Autodesk Inventor part; units mm, degrees
ref_plane "Work Plane5" through (-11.5, 0, 1.25) normal (1, 0, 0) x (0, 0, -1)
ref_plane "Work Plane6" through (-24.25, 0, -17.5) normal (0, 0, 1) x (1, 0, 0)
ref_plane "YZ Plane" through (0, 0, 0) normal (1, 0, 0) x (0, 1, 0)
sketch "Sketch1" plane through (0, 0, 0) normal (0, 1, 0) x (-1, 0, 0)
  line L0 (0, 0) -> (23, 0) construction
  line L1 (23, 0) -> (23, -35) construction
  line L2 (23, -35) -> (0, -35) construction
  line L3 (0, -35) -> (0, 0) construction
  line L4 (23.25, -35.25) -> (23.25, 0.25)
  line L5 (23.25, 0.25) -> (-0.25, 0.25)
  line L6 (-0.25, 0.25) -> (-0.25, -35.25)
  line L7 (-0.25, -35.25) -> (23.25, -35.25)
  line L8 (24.25, 1.25) -> (24.25, -36.25)
  line L9 (24.25, -36.25) -> (-1.25, -36.25)
  line L10 (-1.25, -36.25) -> (-1.25, 1.25)
  line L11 (-1.25, 1.25) -> (24.25, 1.25)
  dimension "d0" = 35
  dimension "d1" = 23
  dimension "d2" = 0.25
  dimension "d3" = 1
extrude "Extrusion1" add sketch "Sketch1" along normal blind 8
sketch "Sketch9" plane through (0.25, 0, 0.25) normal (0, 0, -1) x (-1, 0, 0)
  line L0 (-1, 0) -> (24.5, 0)
  line L1 (24.5, 0) -> (24.5, 8)
  line L2 (-1, 8) -> (24.5, 8)
  line L3 (-1, 0) -> (-1, 8)
  line L4 (0, 0) -> (23.5, 0)
  line L5 (23.5, 0) -> (23.5, 8)
  line L6 (0, 8) -> (23.5, 8)
  line L7 (0, 0) -> (0, 8)
  line L8 (0, 8) -> (3, 8)
  line L9 (24.5, 8) -> (-1, 8)
  line L10 (3, 8) -> (0, 5.5)
  line L11 (0, 0) -> (0, 8)
  line L12 (0, 8) -> (0, 5.5)
  point P0 (0.25, 0)
  point P1 (0, 8)
  dimension "d25" = 3
  dimension "d26" = 2.5
extrude "Extrusion7" add sketch "Sketch9" along normal up to surface (35.5 mm away) contours L7 L2 L10
ref_plane "Work Plane5" through (-11.5, 0, 1.25) normal (1, 0, 0) x (0, 0, -1)
mirror "Mirror4" about plane through (-11.5, 0, 1.25) normal (1, 0, 0) of "Extrusion7"
sketch "Sketch10" plane through (0.25, 0, -35.25) normal (-1, 0, 0) x (0, 0, 1)
  line L0 (-1, 0) -> (36.5, 0)
  line L1 (36.5, 0) -> (36.5, 8)
  line L2 (-1, 8) -> (36.5, 8)
  line L3 (-1, 0) -> (-1, 8)
  line L4 (35.5, 5.5) -> (0, 5.5)
  line L5 (0, 0) -> (0, 5.5)
  line L6 (0, 0) -> (35.5, 0)
  line L7 (35.5, 0) -> (35.5, 5.5)
  line L8 (36.5, 8) -> (-1, 8)
  line L9 (0, 8) -> (3, 8)
  line L10 (0, 0) -> (0, 5.5)
  line L11 (3, 8) -> (0, 5.5)
  line L12 (35.5, 5.5) -> (0, 5.5)
  line L13 (0, 8) -> (0, 5.5)
  point P0 (35.25, 0)
  point P1 (3, 8)
  dimension "d29" = 3
extrude "Extrusion8" add sketch "Sketch10" along normal up to surface (23.5 mm away) contours L13 L2 L11
ref_plane "Work Plane6" through (-24.25, 0, -17.5) normal (0, 0, 1) x (1, 0, 0)
mirror "Mirror5" about plane through (-24.25, 0, -17.5) normal (0, 0, 1) of "Extrusion8"
sketch "Sketch11" plane through (0, 8, 0) normal (0, 1, 0) x (1, 0, 0)
  line L0 (1.25, -1.25) -> (1.25, 36.25)
  line L1 (-24.25, -1.25) -> (1.25, -1.25)
  line L2 (-24.25, 36.25) -> (-24.25, -1.25)
  line L3 (1.25, 36.25) -> (-24.25, 36.25)
  line L4 (-23.25, 35.25) -> (0.25, 35.25)
  line L5 (-23.25, -0.25) -> (-23.25, 35.25)
  line L6 (0.25, -0.25) -> (-23.25, -0.25)
  line L7 (0.25, 35.25) -> (0.25, -0.25)
  point P0 (0, 0)
extrude "Extrusion9" add sketch "Sketch11" along normal blind 3
sketch "Sketch12" plane through (-23.25, 0, -35.25) normal (0, 0, 1) x (1, 0, 0)
  line L0 (23.5, 5.5) -> (0, 5.5)
  line L1 (0, 0) -> (0, 5.5)
  line L2 (0, 0) -> (23.5, 0)
  line L3 (23.5, 0) -> (23.5, 5.5)
  line L4 (0, 5.5) -> (15, 5.5)
  line L5 (15, 5.5) -> (15, 3.5)
  line L6 (15, 3.5) -> (0, 3.5)
  line L7 (0, 3.5) -> (0, 5.5)
  point P0 (23.25, 0)
  point P1 (0, 5.5)
  point P2 (0, 3.5)
  dimension "d34" = 3.5
  dimension "d35" = 2
  dimension "d36" = 15
extrude "Extrusion10" add sketch "Sketch12" along normal blind 3 contours L5 L6 L1 L0
sketch "Sketch13" plane through (0.25, 0, 0.25) normal (0, 0, -1) x (-1, 0, 0)
  line L0 (23.5, 3.5) -> (23.5, 5.5)
  line L1 (8.5, 5.5) -> (23.5, 5.5)
  line L2 (8.5, 3.5) -> (23.5, 3.5)
  line L3 (23.5, 0) -> (23.5, 3.5)
  line L4 (23.5, 0) -> (0, 0)
  line L5 (0, 0) -> (0, 5.5)
  line L6 (0, 5.5) -> (8.5, 5.5)
  line L7 (8.5, 5.5) -> (8.5, 3.5)
  line L8 (7.5, 5.5) -> (7.5, 3.5)
  line L9 (7.5, 3.5) -> (3.5, 3.5)
  line L10 (3.5, 3.5) -> (3.5, 5.5)
  line L11 (3.5, 5.5) -> (7.5, 5.5)
  line L12 (21.5, 5.5) -> (23.5, 5.5)
  line L13 (23.5, 5.5) -> (23.5, 3.5)
  line L14 (23.5, 3.5) -> (21.5, 3.5)
  line L15 (21.5, 3.5) -> (21.5, 5.5)
  point P0 (0.25, 0)
  dimension "d40" = 4
  dimension "d41" = 2
  dimension "d42" = 3.5
  dimension "d49" = 2
extrude "Extrusion11" add sketch "Sketch13" along normal blind 2 contours L2 L15 L1 L0 | L8 L9 L10 L6
sketch "Sketch18" plane through (-23.25, 5.5, -35.25) normal (0, 1, 0) x (1, 0, 0)
  line L0 (16, -35.5) -> (20, -35.5)
  line L1 (20, -35.5) -> (20, -33.5)
  line L2 (16, -33.5) -> (20, -33.5)
  line L3 (16, -35.5) -> (16, -33.5)
  line L4 (0, -35.5) -> (2, -35.5)
  line L5 (2, -35.5) -> (2, -33.5)
  line L6 (0, -33.5) -> (2, -33.5)
  line L7 (0, -33.5) -> (0, -35.5)
  line L8 (15, 0) -> (0, 0)
  line L9 (0, 0) -> (0, -3)
  line L10 (15, -3) -> (0, -3)
  line L11 (15, 0) -> (15, -3)
  point P0 (23.25, -35.25)
extrude "Extrusion14" add sketch "Sketch18" along normal up to surface (2.5 mm away)
sketch "Sketch20" plane through (-23.25, 3.5, -35.25) normal (0, -1, 0) x (1, 0, 0)
  line L0 (0, 35.5) -> (2, 35.5)
  line L1 (0, 33.5) -> (0, 35.5)
  line L2 (2, 33.5) -> (0, 33.5)
  line L3 (2, 35.5) -> (2, 33.5)
  line L4 (16, 35.5) -> (20, 35.5)
  line L5 (16, 35.5) -> (16, 33.5)
  line L6 (20, 33.5) -> (16, 33.5)
  line L7 (20, 35.5) -> (20, 33.5)
  line L8 (15, 0) -> (0, 0)
  line L9 (15, 0) -> (15, 3)
  line L10 (0, 3) -> (15, 3)
  line L11 (0, 0) -> (0, 3)
  point P0 (23.25, 35.25)
extrude "Extrusion16" cut sketch "Sketch20" against normal blind 0.5
sketch "Sketch22" plane through (-23.25, 0, -35.25) normal (0, 0, 1) x (1, 0, 0)
  point P0 (23.25, 0)
sketch "Sketch23" plane through (-23.25, 0, -35.25) normal (0, 0, 1) x (1, 0, 0)
  point P0 (23.25, 0)
properties part number "sensorCover"
The model under review builds one solid part; all positions refer to its coordinate system, in mm. A direction names the side the tool comes from. Give positions to 0.01 mm unless a question says otherwise; leave off trailing zeros. Write each loop counter-clockwise with the first axis right and the second up, starting at its lowest first coordinate (ties: lowest second). Pieces come first, ordered by that corner, then holes. Notation, with made-up numbers: M 24,75.5 L 54,75.5 A14 ccw 54,94.5 Z; hole C 88.25,41 d2. An arc over 180 degrees is marked long. One line per question, with ' | ' between items. Start each with the question number.
Item 1: We need section A-A on z = -7. Write out the cut boundary in (x, y).
Item 2: Wall thickness on line 1 (X direction, y = 0.75, z = -1); line 2 (Z direction, x = -7.5, y = 2.5); line 3 (X direction, y = 4.5, z = -1): over which ranges is each line inside the solid? List them lowest first. Write a range as from..to.
Item 3: We need section C-C on x = -16. Write out the cut boundary in (y, z), plus the area to 4 significant figures.
Item 4: Draft analysis for pull direction X (two halves, no side actions). For faces 3 (the flat face through (-24.25, 5, -18)), 4 (the flat face through (1.25, 5, -17)), 5 (the flat face through (-11, 2, -35.25)), state which applies: released by +X, released by -X, zero draft, split by the parting line, or undercut.
Item 5: We need section D-D on y = 4.5. Write out the cut boundary in (x, z).
Item 6: For faces 1 (the flat face through (-22, 4, -1)), 2 (the flat face through (-23.25, 9, -17)), list the 3-axis set-ups (+Z, -Z, +X, -X, +Y, -Y) from which the entire face can be reached by the end or side of a thin tool; tool diameter is ignored.
Item 7: We need section B-B on y = 9.75. Write out the cut boundary in (x, z).
Item 8: For pin 1 (1.6 mm diameter, centred on x = -5, z = -1, fed in from -Y); pin 2 (5 mm diameter, centred on x = -20, z = -13.5, fed in from -Y) (3 decimals), all flat-tipped, find the tip position at first contact; note any pin that passes through.
Results found:
1) outline: M -24.25,0 L -23.25,0 L -23.25,5.5 L -20.25,8 L -23.25,8 L -23.25,11 L -24.25,11 Z; M -2.75,8 L 0.25,5.5 L 0.25,0 L 1.25,0 L 1.25,11 L 0.25,11 L 0.25,8 Z
2) line 1: x = -24.25..-23.25, 0.25..1.25 | line 2: z = -36.25..-35.25, 0.25..1.25 | line 3: x = -24.25..-21.25, -7.25..-3.25, 0.25..1.25
3) outline: M 0,-36.25 L 11,-36.25 L 11,-35.25 L 8,-35.25 L 8,-32.25 L 4,-32.25 L 4,-35.25 L 0,-35.25 Z; M 0,0.25 L 5.5,0.25 L 8,-2.75 L 8,0.25 L 11,0.25 L 11,1.25 L 0,1.25 Z | area: 37.75 mm2
4) face 3: released by -X | face 4: released by +X | face 5: undercut
5) outline: M -24.25,-36.25 L 1.25,-36.25 L 1.25,1.25 L -24.25,1.25 Z; hole M -23.25,-32.25 L -8.25,-32.25 L -8.25,-35.25 L 0.25,-35.25 L 0.25,0.25 L -3.25,0.25 L -3.25,-1.75 L -7.25,-1.75 L -7.25,0.25 L -21.25,0.25 L -21.25,-1.75 L -23.25,-1.75 Z
6) face 1: -Y | face 2: +Y
7) outline: M -24.25,-36.25 L 1.25,-36.25 L 1.25,1.25 L -24.25,1.25 Z; hole M -23.25,-35.25 L 0.25,-35.25 L 0.25,0.25 L -23.25,0.25 Z
8) pin 1: stops at y = 4 | pin 2: stops at y = 6.125
